For this review, take the finished solid that the model builds, in its own axes (mm). Round coordinates to 2 decimals unless told otherwise and drop trailing zeros. Order: outer loops, then holes, each group sorted by start corner. A loop starts at its lowest first (then second) coordinate and runs counter-clockwise, first axis right, second up. Notation, with made-up numbers: (23.5, 65) -> (70.5, 65) arc R17 cw to (70.5, 77) -> close; hole circle Ø1 at (65.25, 53.25). An arc over 180 degrees is marked (long way). Use a Markdown table: item, result. Add a question column.
1) Consider section A-A (z = 47.5). State the section outline as (x, y) points (3 decimals), plus the area to 3 significant figures.
2) Wall thickness on line 1 along Z through (x, y) = (-68, 1.95); line 2 along Z through (x, y) = (-85, 1.3); line 3 along X through (y, z) = (0.3, 55): over which ranges is each line inside the solid? List them lowest first. Write a range as [from, to].
3) Consider section C-C (y = 1.85). Give the number of separate pieces and of enclosed holes in the cut face, plus the area to 3 significant figures.
4) Consider section B-B (x = -2.5). State the section outline as (y, z) points, plus the area to 3 significant figures.
5) Clearance check with a flat-ended pin moving along its axis: P1, Ø18.5, axis at x = 0, z = 52.5, coming from the +Y side. State where the tip first meets the part, or that it passes through.
```python
from build123d import *

# Parameters (mm, degrees)
SKETCH1_W           = 210
SKETCH1_H           = 230
BOSS_EXTRUDE1_DEPTH = 3
FILLET1_R           = 10
SKETCH2_R           = 1.7
CUT_EXTRUDE1_DEPTH  = 3
SKETCH3_R           = 4
CUT_EXTRUDE2_DEPTH  = 176.025712397
SKETCH4_R           = 8
CUT_EXTRUDE3_DEPTH  = 176.025712397
CUT_EXTRUDE4_DEPTH  = 176.025712397
SKETCH6_R           = 4
SKETCH6_R_2         = 1.7
CUT_EXTRUDE5_DEPTH  = 176.025712397


with BuildPart() as part:
    # Sketch1 → Boss-Extrude1 (new body)
    with BuildSketch(Plane(origin=(0, 0, 0), x_dir=(1, 0, 0), z_dir=(0, 1, 0))):
        with Locations((0, 25)):
            Rectangle(SKETCH1_W, SKETCH1_H)
    extrude(amount=BOSS_EXTRUDE1_DEPTH)

    # Fillet1
    fillet1_edges = [part.edges().sort_by_distance(p)[0] for p in [
        (105, 1.5, 90),
        (-105, 1.5, 90),
        (-105, 1.5, -140),
        (105, 1.5, -140),
    ]]
    fillet(fillet1_edges, radius=FILLET1_R)

    # Sketch2 → Cut-Extrude1 (cut)
    with BuildSketch(Plane(origin=(0, 3, 0), x_dir=(1, 0, 0), z_dir=(0, 1, 0))):
        with Locations(Location((-82, 120, 0), (0, 0, 270))):
            Circle(SKETCH2_R)
        with Locations(Location((-68, 120, 0), (0, 0, 270))):
            Circle(SKETCH2_R)
        with Locations(Location((68, 120, 0), (0, 0, 270))):
            Circle(SKETCH2_R)
        with Locations(Location((82, 120, 0), (0, 0, 270))):
            Circle(SKETCH2_R)
        with Locations(Location((-82, -75, 0), (0, 0, 270))):
            Circle(SKETCH2_R)
        with Locations(Location((-68, -75, 0), (0, 0, 270))):
            Circle(SKETCH2_R)
        with Locations(Location((68, -75, 0), (0, 0, 270))):
            Circle(SKETCH2_R)
        with Locations(Location((82, -75, 0), (0, 0, 270))):
            Circle(SKETCH2_R)
        with Locations(Location((-54, -75, 0), (0, 0, 270))):
            Circle(SKETCH2_R)
        with Locations(Location((54, -75, 0), (0, 0, 270))):
            Circle(SKETCH2_R)
        with Locations(Location((-40, -75, 0), (0, 0, 270))):
            Circle(SKETCH2_R)
        with Locations(Location((40, -75, 0), (0, 0, 270))):
            Circle(SKETCH2_R)
    extrude(amount=-CUT_EXTRUDE1_DEPTH, mode=Mode.SUBTRACT)

    # Sketch3 → Cut-Extrude2 (cut, through all)
    with BuildSketch(Plane(origin=(0, 3, 0), x_dir=(1, 0, 0), z_dir=(0, 1, 0))):
        with Locations(Location((40, 65, 0), (0, 0, 270))):
            Circle(SKETCH3_R)
    extrude(amount=-CUT_EXTRUDE2_DEPTH, mode=Mode.SUBTRACT)

    # Sketch4 → Cut-Extrude3 (cut, through all)
    with BuildSketch(Plane(origin=(0, 3, 0), x_dir=(1, 0, 0), z_dir=(0, 1, 0))):
        with Locations(Location((0, -52.5, 0), (0, 0, 270))):
            Circle(SKETCH4_R)
    extrude(amount=-CUT_EXTRUDE3_DEPTH, mode=Mode.SUBTRACT)

    # Sketch5 → Cut-Extrude4 (cut, through all)
    with BuildSketch(Plane(origin=(0, 3, 0), x_dir=(1, 0, 0), z_dir=(0, 1, 0))):
        with BuildLine():
            Line((67.757117203, -10), (67.757117203, -50))
            ThreePointArc((67.757117203, -50), (60.791955234, -56.965161969), (53.826793265, -50))
            Line((53.826793265, -50), (53.826793265, -10))
            ThreePointArc((53.826793265, -10), (60.791955234, -3.034838031), (67.757117203, -10))
        make_face()
        with BuildLine():
            Line((-80, -43.92126235), (-60, -43.92126235))
            ThreePointArc((-60, -43.92126235), (-51.42126235, -52.5), (-60, -61.07873765))
            Line((-60, -61.07873765), (-80, -61.07873765))
            ThreePointArc((-80, -61.07873765), (-88.57873765, -52.5), (-80, -43.92126235))
        make_face()
    extrude(amount=-CUT_EXTRUDE4_DEPTH, mode=Mode.SUBTRACT)

    # Sketch6 → Cut-Extrude5 (cut, through all)
    with BuildSketch(Plane(origin=(0, 3, 0), x_dir=(1, 0, 0), z_dir=(0, 1, 0))):
        with Locations(Location((-56.482041844, 24.314281351, 0), (0, 0, 270))):
            Circle(SKETCH6_R)
        with Locations(Location((-84.211086261, 107.143726059, 0), (0, 0, 270))):
            Circle(SKETCH6_R_2)
        with Locations(Location((-54.215528573, 106.627471285, 0), (0, 0, 270))):
            Circle(SKETCH6_R_2)
        with Locations(Location((-56.452632591, -23.353278696, 0), (0, 0, 270))):
            Circle(SKETCH6_R_2)
        with Locations(Location((-86.448190279, -22.837023922, 0), (0, 0, 270))):
            Circle(SKETCH6_R_2)
    extrude(amount=-CUT_EXTRUDE5_DEPTH, mode=Mode.SUBTRACT)


solid = part.part
```
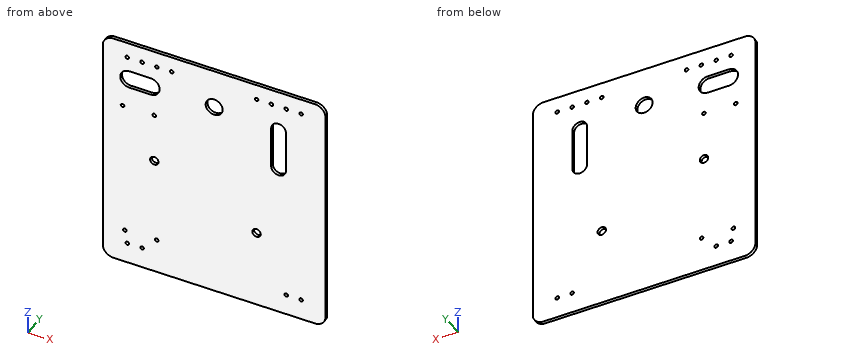
Results list:
| question | item | result |
|---|---|---|
| 1 | outline | (-105, 0) -> (-86.971, 0) -> (-86.971, 3) -> (-105, 3) -> close; (-53.029, 0) -> (-6.245, 0) -> (-6.245, 3) -> (-53.029, 3) -> close; (6.245, 0) -> (53.827, 0) -> (53.827, 3) -> (6.245, 3) -> close; (67.757, 0) -> (105, 0) -> (105, 3) -> (67.757, 3) -> close |
| 1 | area | 449 mm2 |
| 2 | line 1 | [-140, -121.7], [-118.3, 43.92], [61.08, 73.3], [76.7, 90] |
| 2 | line 2 | [-140, -108.65], [-105.64, 21.95], [23.73, 45.53], [59.47, 90] |
| 2 | line 3 | [-105, -88.21], [-51.79, -7.6], [7.6, 55.94], [65.64, 105] |
| 3 | separate pieces | 1 |
| 3 | enclosed holes | 21 |
| 3 | area | 46,500 mm2 |
| 4 | outline | (0, -140) -> (3, -140) -> (3, 44.9) -> (0, 44.9) -> close; (0, 60.1) -> (3, 60.1) -> (3, 90) -> (0, 90) -> close |
| 4 | area | 644 mm2 |
| 5 | P1 | y = 3 |
